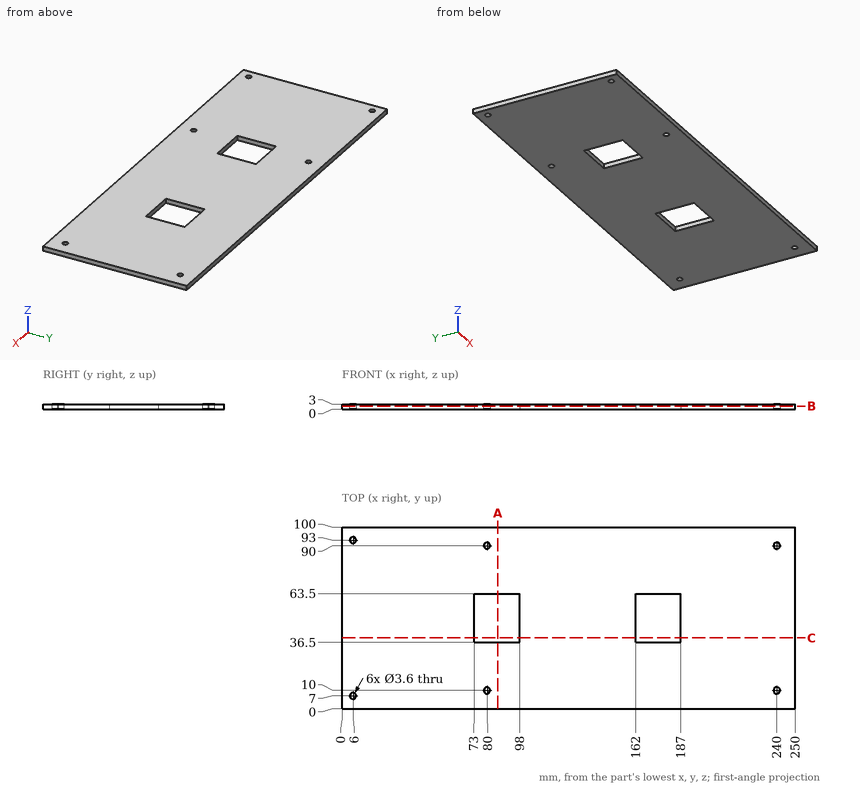
Source: three-view drawing plus pictorial views. Frame: mm from the lowest corner of the part. Round coordinates to 2 decimals unless told otherwise and drop trailing zeros. Order: outer loops, then holes, each group sorted by start corner. A loop starts at its lowest first (then second) coordinate and runs counter-clockwise, first axis right, second up. Notation, with made-up numbers: M 1,42.5 L 22,42.5 A24 ccw 22,66.5 Z; hole C 87,41.5 d3. An arc over 180 degrees is marked long. One line per item, written item: value.
(1) Cut plane C-C (y = 39). Return the cut outline in (x, z), and give its area (3 significant figures).
Result sheet:
outline: M 0,0 L 73,0 L 73,3 L 0,3 Z; M 98,0 L 162,0 L 162,3 L 98,3 Z; M 187,0 L 250,0 L 250,3 L 187,3 Z
area: 600 mm2
(2) Cut plane B-B (z = 1.85). Give the number of separate pieces and of enclosed holes in the cut face, and give its area (3 significant figures).
Result sheet:
separate pieces: 1
enclosed holes: 8
area: 23,600 mm2
(3) Cut plane A-A (x = 86). Return the cut outline in (y, z), and give its area (3 significant figures).
Result sheet:
outline: M 0,0 L 36.5,0 L 36.5,3 L 0,3 Z; M 63.5,0 L 100,0 L 100,3 L 63.5,3 Z
area: 219 mm2
(4) Line query: probe 1 along X at (y, z) = (90, 1.6); probe 2 along X at (y, z) = (53, 0.2); probe 3 along Y at (x, z) = (80, 0.7). Output: solid intervals per line, ascending. Write a range as [from, to].
Result sheet:
probe 1: [0, 78.2], [81.8, 238.2], [241.8, 250]
probe 2: [0, 73], [98, 162], [187, 250]
probe 3: [0, 8.2], [11.8, 36.5], [63.5, 88.2], [91.8, 100]
